Part model, mm, in its own coordinate system. Face numbers are marked on the shaded views. A direction names the side the tool comes from. Coordinates: 2 decimals unless noted, no trailing zeros. Write each loop counter-clockwise with the first axis right and the second up, starting at its lowest first coordinate (ties: lowest second). Pieces come first, ordered by that corner, then holes. Notation, with made-up numbers: M 11.25,74.25 L 58.25,74.25 A7 ccw 58.25,83.25 Z; hole C 9,5 d6. An arc over 180 degrees is marked long. Use a Markdown table: item, result. Add a question column.
Q1. Tool access for the marked faces 4 and 5: list every direction of +Z, -Z, +X, -X, +Y, -Y with a clear straight run to the whole face (end or side of a thin tool).
Q2. Slice it at A-A on x = 0. Write the cut outline in (y, z), then the cut area to 3 significant figures.
Q3. Slice it at C-C on z = 1.75. Write the cut outline in (x, y).
Q4. Slice it at D-D on x = -1.7. Write the cut outline in (y, z).
Q5. Slice it at B-B on y = 29.5. Write the cut outline in (x, z).
Q6. Wall check: L1, parallel to Y at x = 0.8, z = -1.4; L2, parallel to X at y = 8, z = 1.65; L3, parallel to Z at x = -1.5, y = 8. Give the ranges that are in metal, low to high. Write a range as from..to.
Q7. Mould opens along Z. For the marked faces 1, 2 and 3 say: released by +Z, released by -Z, zero draft, split by the parting line, or undercut.
Q8. Pin check, flat tips, straight feed: pin 1 Ø1 at (x, z) = (1, 1.5) entering from +Y; pin 2 Ø1 at (y, z) = (10.5, -1.5) entering from +X. Stop position of each tip, or through.
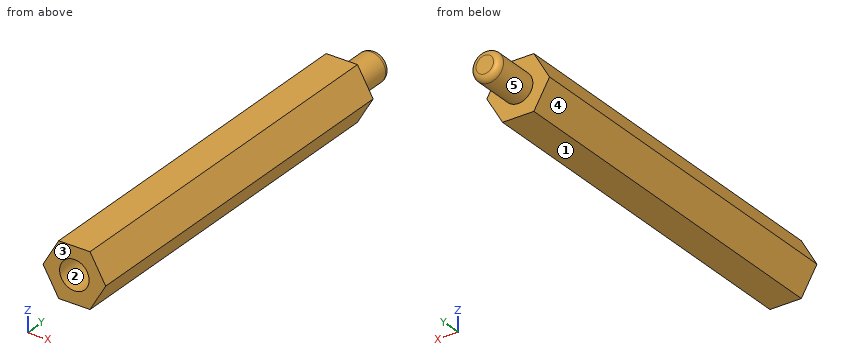
from build123d import *

# Parameters (mm, degrees)
SALIENTE_EXTRUIR1_DEPTH = 32
CROQUIS_SUPERIOR_R      = 1.24
SALIENTE_EXTRUIR2_DEPTH = 4
REDONDEO1_R             = 0.5
CROQUIS_INFERIOR_R      = 1.25
CORTAR_EXTRUIR1_DEPTH   = 4


with BuildPart() as part:
    # Croquis base → Saliente-Extruir1 (new body)
    with BuildSketch(Plane(origin=(0, 0, 0), x_dir=(1, 0, 0), z_dir=(0, 1, 0))):
        Polygon((2.655811238, 0), (1.327905619, 2.3), (-1.327905619, 2.3), (-2.655811238, 0), (-1.327905619, -2.3), (1.327905619, -2.3), align=None)
    extrude(amount=SALIENTE_EXTRUIR1_DEPTH)

    # Croquis Superior → Saliente-Extruir2 (add)
    with BuildSketch(Plane(origin=(0, 32, 0), x_dir=(1, 0, 0), z_dir=(0, 1, 0))):
        with Locations(Location((0, 0, 0), (0, 0, 270))):
            Circle(CROQUIS_SUPERIOR_R)
    extrude(amount=SALIENTE_EXTRUIR2_DEPTH)

    # Redondeo1
    redondeo1_edges = [part.edges().sort_by_distance(p)[0] for p in [
        (0, 36, -1.24),
    ]]
    fillet(redondeo1_edges, radius=REDONDEO1_R)

    # Croquis inferior → Cortar-Extruir1 (cut)
    with BuildSketch(Plane(origin=(0, 0, 0), x_dir=(-1, 0, 0), z_dir=(0, -1, 0))):
        with Locations(Location((0, 0, 0), (0, 0, 90))):
            Circle(CROQUIS_INFERIOR_R)
    extrude(amount=-CORTAR_EXTRUIR1_DEPTH, mode=Mode.SUBTRACT)


solid = part.part
Recorded:
| question | item | result |
|---|---|---|
| 1 | face 4 | -Z, -X, +Y, -Y |
| 1 | face 5 | +Y |
| 2 | outline | M 0,-2.3 L 32,-2.3 L 32,-1.24 L 35.5,-1.24 A0.5 ccw 36,-0.74 L 36,0.74 A0.5 ccw 35.5,1.24 L 32,1.24 L 32,2.3 L 0,2.3 L 0,1.25 L 4,1.25 L 4,-1.25 L 0,-1.25 Z |
| 2 | area | 147 mm² |
| 3 | outline | M -1.65,0 L 1.65,0 L 1.65,32 L -1.65,32 Z |
| 4 | outline | M 0,-1.66 L 32,-1.66 L 32,1.66 L 0,1.66 Z |
| 5 | outline | M -2.66,0 L -1.33,-2.3 L 1.33,-2.3 L 2.66,0 L 1.33,2.3 L -1.33,2.3 Z |
| 6 | L1 | 0..32 |
| 6 | L2 | -1.7..1.7 |
| 6 | L3 | -2..2 |
| 7 | face 1 | released by -Z |
| 7 | face 2 | undercut |
| 7 | face 3 | zero draft |
| 8 | pin 1 | y = 32 |
| 8 | pin 2 | x = 2.08 |
